from build123d import *

# Parameters (mm, degrees)
CORTAR_EXTRUIR1_DEPTH      = 10
CORTAR_EXTRUIR1_DEPTH_BACK = 10
CROQUIS3_R                 = 4
CHAFL_N1_SIZE              = 0.366025404


with BuildPart() as part:
    # Croquis1 → Revolución1 (revolve)
    with BuildSketch(Plane.XY):
        with BuildLine():
            Line((0, 0), (0, -8))
            ThreePointArc((0, -8), (8, 0), (0, 8))
            Line((0, 8), (0, 0))
        make_face()
    revolve(axis=Axis((0, -8, 0), (0, 1, 0)))

    # Croquis3 → Cortar-Extruir1 (cut, two sides: drawn at the far end of the back side and taken through both)
    with BuildSketch(Plane(origin=(0, 0, 0), x_dir=(1, 0, 0), z_dir=(0, 1, 0)).offset(-CORTAR_EXTRUIR1_DEPTH_BACK)):
        with Locations(Location((0, 0, 0), (0, 0, 180))):
            Circle(CROQUIS3_R)
    extrude(amount=CORTAR_EXTRUIR1_DEPTH + CORTAR_EXTRUIR1_DEPTH_BACK, mode=Mode.SUBTRACT)

    # Chaflán1
    # the kernel refuses this chamfer: 0.5, 0.366025404 mm, written as the material it takes off along each edge
    with BuildSketch(Plane(origin=(0, -6.92820323, 0), x_dir=(-1, 0, 0), z_dir=(0, 0, -1))) as chafl_n1_piece_1:
        with BuildLine():
            Line((4.412889217, 0.255392072), (4, CHAFL_N1_SIZE))
            Line((4, CHAFL_N1_SIZE), (4, 0))
            ThreePointArc((4, 0), (4.214206629, 0.128169224), (4.412889217, 0.255392072))
        make_face()
    revolve(axis=Axis((0, -6.92820323, 0), (0, 1, 0)), revolution_arc=180, mode=Mode.SUBTRACT)
    with BuildSketch(Plane(origin=(0, 6.92820323, 0), x_dir=(-1, 0, 0), z_dir=(0, 0, 1))) as chafl_n1_piece_2:
        with BuildLine():
            Line((4.412889217, 0.255392072), (4, CHAFL_N1_SIZE))
            Line((4, CHAFL_N1_SIZE), (4, 0))
            ThreePointArc((4, 0), (4.214206629, 0.128169224), (4.412889217, 0.255392072))
        make_face()
    revolve(axis=Axis((0, 6.92820323, 0), (0, -1, 0)), revolution_arc=180, mode=Mode.SUBTRACT)
    with BuildSketch(Plane(origin=(0, 6.92820323, 0), x_dir=(1, 0, 0), z_dir=(0, 0, -1))) as chafl_n1_piece_3:
        with BuildLine():
            Line((4.412889217, 0.255392072), (4, CHAFL_N1_SIZE))
            Line((4, CHAFL_N1_SIZE), (4, 0))
            ThreePointArc((4, 0), (4.214206629, 0.128169224), (4.412889217, 0.255392072))
        make_face()
    revolve(axis=Axis((0, 6.92820323, 0), (0, -1, 0)), revolution_arc=180, mode=Mode.SUBTRACT)
    with BuildSketch(Plane(origin=(0, -6.92820323, 0), x_dir=(1, 0, 0), z_dir=(0, 0, 1))) as chafl_n1_piece_4:
        with BuildLine():
            Line((4.412889217, 0.255392072), (4, CHAFL_N1_SIZE))
            Line((4, CHAFL_N1_SIZE), (4, 0))
            ThreePointArc((4, 0), (4.214206629, 0.128169224), (4.412889217, 0.255392072))
        make_face()
    revolve(axis=Axis((0, -6.92820323, 0), (0, 1, 0)), revolution_arc=180, mode=Mode.SUBTRACT)


solid = part.part
Read the model definition and answer for the solid it produces. Units are mm, in the model's axes. Give positions to 0.01 mm unless a question says otherwise; leave off trailing zeros. Loops run counter-clockwise (first coordinate to the right, second up) from the corner with the lowest first, then second, coordinate; pieces in that order, holes last. Notation, with made-up numbers: (-24.75, 65.25) - (30.25, 65.25) arc R20 ccw to (30.25, 100.25) - close; hole circle Ø7 at (-16, 21.25). An arc over 180 degrees is marked (long way). Answer as CSV lines item,"result". Start each with the question number.
1) Find section B-B (z = 0). Write down the section's boundary in (x, y), then the cut area to 3 significant figures.
2) Straight lines are drawn through the part: L1, parallel to X at y = -1.75, z = -0.25; L2, parallel to X at y = 3, z = 1.5; L3, parallel to Z at x = -0.25, y = -4.5. For each, find the intervals that lie inside material, in ascending order. Write a range as from..to.
3) Find section D-D (x = 5.25). Write down the section's boundary in (y, z), then the cut area to 3 significant figures.
4) Each of these flat-tipped pins is pushed along its axis until it touches: pin 1 Ø3 at (x, y) = (-4.5, 0) entering from -Z; pin 2 Ø3 at (x, y) = (5.5, -4.5) entering from -Z; pin 3 Ø9 at (x, z) = (0, 0) entering from +Y; pin 4 Ø2 at (x, y) = (3, -3.5) entering from -Z. Where does it stop, or does it pass through?
5) Find section C-C (y = -4.75). Write down the section's boundary in (x, z), then the cut area to 3 significant figures.
6) Find section A-A (x = 0). Write down the section's boundary in (y, z).
Findings below:
1,outline,"(-4.41, -6.67) - (-4, -6.56) - (-4, 6.56) - (-4.41, 6.67) arc R8 ccw to start; (4, -6.56) - (4.41, -6.67) arc R8 ccw to (4.41, 6.67) - (4, 6.56) - close"
1,area,"78.3 mm^2"
2,L1,"-7.8..-3.99, 3.99..7.8"
2,L2,"-7.26..-3.71, 3.71..7.26"
2,L3,"-6.61..-3.99, 3.99..6.61"
3,outline,"circle Ø12.07 at (0, 0)"
3,area,"114 mm^2"
4,pin 1,"z = -7.42"
4,pin 2,"z = -5.71"
4,pin 3,"y = 6.67"
4,pin 4,"z = -7.14"
5,outline,"circle Ø12.87 at (0, 0); hole circle Ø8 at (0, 0)"
5,area,"79.9 mm^2"
6,outline,"(-6.67, -4.41) arc R8 ccw to (6.67, -4.41) - (6.56, -4) - (-6.56, -4) - close; (-6.67, 4.41) - (-6.56, 4) - (6.56, 4) - (6.67, 4.41) arc R8 ccw to start"
